from build123d import *

# Parameters (mm, degrees)
F0_R     = 11.0236
F1_DEPTH = 6.35
F3_DEPTH = 6.35


with BuildPart() as f1:
    # F0 (on Top) → F1 (new body)
    with BuildSketch(Plane.XY):
        Polygon((-48.3935, -27.94), (48.3935, -27.94), (0, 55.88), align=None)
        with Locations((-22.392992, -12.9286)):
            Circle(F0_R, mode=Mode.SUBTRACT)
        with Locations((22.392992, -12.9286)):
            Circle(F0_R, mode=Mode.SUBTRACT)
        Circle(F0_R, mode=Mode.SUBTRACT)
        with Locations((0, 25.8572)):
            Circle(F0_R, mode=Mode.SUBTRACT)
    extrude(amount=F1_DEPTH)

    # F2 (on face) → F3 (cut)
    with BuildSketch(Plane.XY.offset(6.35)):
        Polygon((-9.740262, 11.409466), (-19.889175, 11.883968), (-15.225649, 2.8575), align=None)
        Polygon((5.138157, -14.614549), (-5.010757, -14.140047), (-0.347231, -23.166515), align=None)
        Polygon((10.087492, 11.757049), (14.751018, 2.730581), (20.236406, 11.282547), align=None)
    extrude(amount=-F3_DEPTH, mode=Mode.SUBTRACT)


solid = f1.part
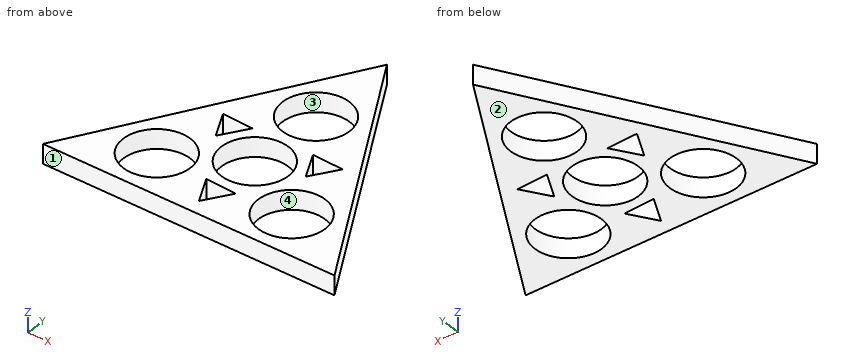
Build history of the part. All positions in model axes, mm. Face numbers are marked on the shaded views. Coordinates: 2 decimals unless noted, no trailing zeros. Order: outer loops, then holes, each group sorted by start corner. A loop starts at its lowest first (then second) coordinate and runs counter-clockwise, first axis right, second up. Notation, with made-up numbers: (89, 46.5) - (147, 46.5) arc R21 ccw to (147, 60.5) - close; hole circle Ø2 at (57, 71.25). An arc over 180 degrees is marked (long way). Write item = value, one per line. Start each with the question number.
1) Flat gauge pins, fed straight in: pin 1 Ø3 at (y, z) = (21.5, 4) entering from -X; pin 2 Ø17.5 at (x, y) = (0, 25.86) entering from +Z; pin 3 Ø1.5 at (x, z) = (-26, 5.5) entering from +Y. Where does each tip first touch, or does it go through?
2) Wall check: line 1 along X through (y, z) = (-13, 0.5); line 2 along Y through (x, z) = (20, 1.5); line 3 along Y through (x, z) = (21, 4.5). Give the ranges that are in metal, low to high. Write a range as from..to.
3) Saw through at B-B on x = -14. Write the cut outline in (y, z), then the cut area to 3 significant figures.
4) Two-plate mould, pull along Y, no slides. Class the marked faces 1, 2, 3 and 4: pulls with the +Y half, pulls with the -Y half, needs draft (parallel to the pull), parting line crosses it, or undercut.
5) Saw through at A-A on y = 5.5. Write the cut outline in (x, z).
6) Saw through at D-D on x = -27. Write the cut outline in (y, z).
7) Saw through at C-C on z = 5. Write the cut outline in (x, y).
From the geometry:
q1.pin_1 = -20.72
q1.pin_2 = through
q1.pin_3 = 12.15
q2.line_1 = -39.77..-33.42, -11.37..11.37, 33.42..39.77
q2.line_2 = -27.94..-23.69, -2.17..10.91, 11.29..21.24
q2.line_3 = -27.94..-23.86, -1.99..19.51
q3.outline = (-27.94, 0) - (-20.08, 0) - (-20.08, 6.35) - (-27.94, 6.35) - close; (-5.78, 0) - (4.77, 0) - (4.77, 6.35) - (-5.78, 6.35) - close; (11.61, 0) - (31.63, 0) - (31.63, 6.35) - (11.61, 6.35) - close
q3.area = 244 mm^2
q4.face_1 = pulls with the -Y half
q4.face_2 = needs draft
q4.face_3 = undercut
q4.face_4 = undercut
q5.outline = (-29.09, 0) - (-16.59, 0) - (-16.59, 6.35) - (-29.09, 6.35) - close; (-13.53, 0) - (-9.55, 0) - (-9.55, 6.35) - (-13.53, 6.35) - close; (9.55, 0) - (13.32, 0) - (13.32, 6.35) - (9.55, 6.35) - close; (16.53, 0) - (29.09, 0) - (29.09, 6.35) - (16.53, 6.35) - close
q6.outline = (-27.94, 0) - (-22.94, 0) - (-22.94, 6.35) - (-27.94, 6.35) - close; (-2.91, 0) - (9.11, 0) - (9.11, 6.35) - (-2.91, 6.35) - close
q7.outline = (-48.39, -27.94) - (48.39, -27.94) - (0, 55.88) - close; hole circle Ø22.05 at (-22.39, -12.93); hole (-19.89, 11.88) - (-15.23, 2.86) - (-9.74, 11.41) - close; hole circle Ø22.05 at (0, 0); hole circle Ø22.05 at (0, 25.86); hole (-5.01, -14.14) - (-0.35, -23.17) - (5.14, -14.61) - close; hole (10.09, 11.76) - (14.75, 2.73) - (20.24, 11.28) - close; hole circle Ø22.05 at (22.39, -12.93)
